Geometry: see drawing. Coordinates: mm, zero at the bounding-box minimum. A direction names the side the tool comes from. Coordinates: 2 decimals unless noted, no trailing zeros. Order: outer loops, then holes, each group sorted by start corner. A loop starts at its lowest first (then second) coordinate and runs counter-clockwise, first axis right, second up. Notation, with made-up numbers: (14.5, 34) -> (46.5, 34) arc R25 ccw to (46.5, 66) -> close; hole circle Ø6 at (26.25, -7.75). An arc over 180 degrees is marked (long way). Write each question's results on one line, items separated by ' | '.
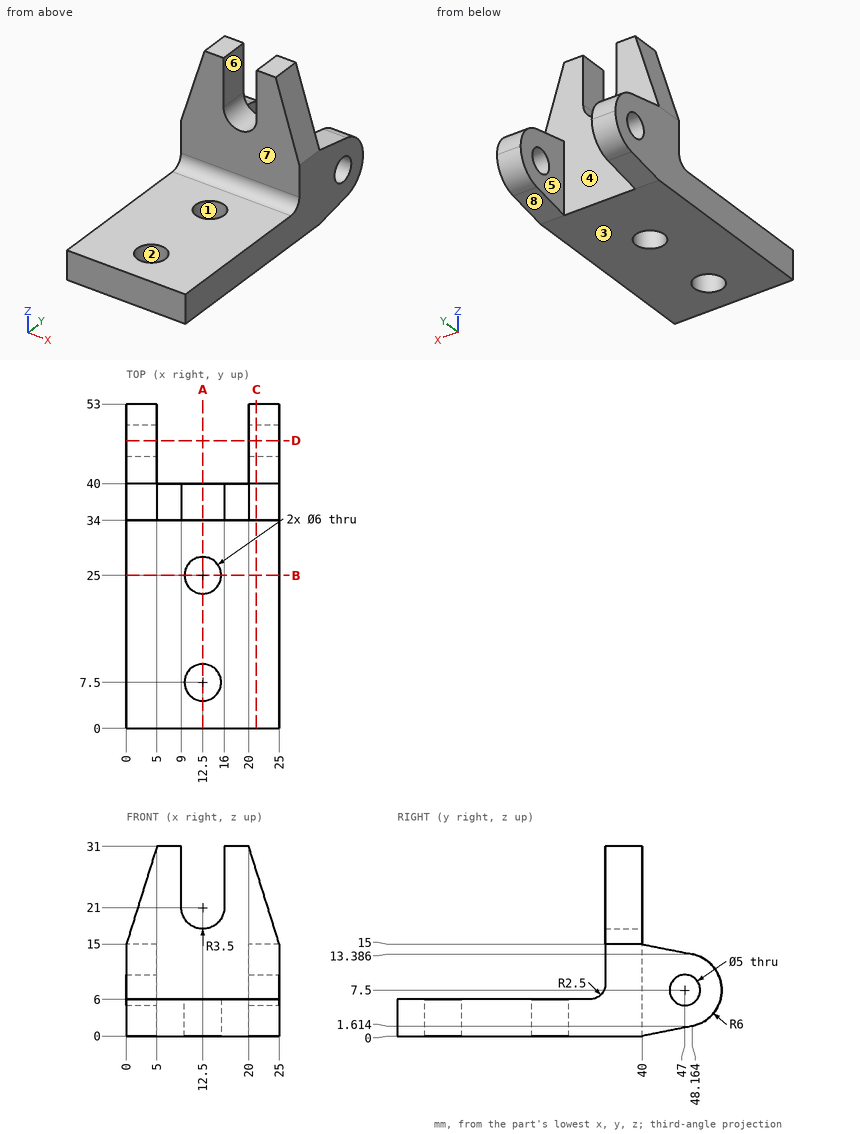
(1) Cut plane B-B, the plane y = 25. Return loops of the section in (x, z).
Return value:
outline: (0, 0) -> (9.5, 0) -> (9.5, 6) -> (0, 6) -> close; (15.5, 0) -> (25, 0) -> (25, 6) -> (15.5, 6) -> close
(2) Pin query (flat end, axial travel): P1, Ø6.5, axis at y = 35.5, z = 23.5, coming from the +X side; P2, Ø7, axis at x = 10, z = 23, coming from the -Y side; P3, Ø10, axis at x = 17, y = 10, coming from the +Z side. Return the tip coordinate at first contact, or that it passes through.
Return value:
P1: x = 23.36 | P2: y = 34 | P3: z = 6
(3) Cut plane A-A, the plane x = 12.5. Return loops of the section in (y, z).
Return value:
outline: (0, 0) -> (4.5, 0) -> (4.5, 6) -> (0, 6) -> close; (10.5, 0) -> (22, 0) -> (22, 6) -> (10.5, 6) -> close; (28, 0) -> (40, 0) -> (40, 17.5) -> (34, 17.5) -> (34, 8.5) arc R2.5 cw to (31.5, 6) -> (28, 6) -> close
(4) Cut plane C-C, the plane x = 21.25. Return loops of the section in (y, z).
Return value:
outline: (0, 0) -> (40, 0) -> (48.16, 1.61) arc R6 ccw to (53, 7.5) arc R6 ccw to (48.16, 13.39) -> (40, 15) -> (40, 27) -> (34, 27) -> (34, 8.5) arc R2.5 cw to (31.5, 6) -> (0, 6) -> close; hole circle Ø5 at (47, 7.5)
(5) Mould query, pull axis Y, two halves, no side actions, for the marked faces 1, 2, 3 and 4. Classes: +Y half, -Y half, draft (parallel to the pull), parting line (faces both ways), or undercut.
Return value:
face 1: undercut | face 2: undercut | face 3: draft | face 4: +Y half
(6) Reachability of the marked faces 5, 6, 7 and 8 from +Z, -Z, +X, -X, +Y, -Y: full face, straight path, thin tool, end or side. Return the list, or none.
Return value:
face 5: +Z, -Z, +Y | face 6: +Z, +Y, -Y | face 7: +Z, +X, -X, -Y | face 8: -Z, +X, -X, +Y
(7) Line query: line 1 along Y through (x, z) = (12.5, 4.8); line 2 along X through (y, z) = (50, 6); line 3 along Y through (x, z) = (12.5, 10). Output: solid intervals per line, ascending. Write a range as from..to.
Return value:
line 1: 0..4.5, 10.5..22, 28..40 | line 2: 0..5, 20..25 | line 3: 34..40
(8) Cut plane D-D, the plane y = 47. Return loops of the section in (x, z).
Return value:
outline: (0, 1.38) -> (5, 1.38) -> (5, 5) -> (0, 5) -> close; (0, 10) -> (5, 10) -> (5, 13.62) -> (0, 13.62) -> close; (20, 1.38) -> (25, 1.38) -> (25, 5) -> (20, 5) -> close; (20, 10) -> (25, 10) -> (25, 13.62) -> (20, 13.62) -> close
